Could you check a few things on this drawing? It's one solid part, dimensions in mm from its lowest x, y, z. Give positions to 0.01 mm unless a question says otherwise; leave off trailing zeros. Order: outer loops, then holes, each group sorted by start corner. A loop starts at its lowest first (then second) coordinate and runs counter-clockwise, first axis right, second up. Notation, with made-up numbers: M 59.5,-39 L 110.5,-39 A26 cw 110.5,-7 Z; hole C 17.5,38.5 d2. An arc over 180 degrees is marked long. Use one line per item in the form item = value.
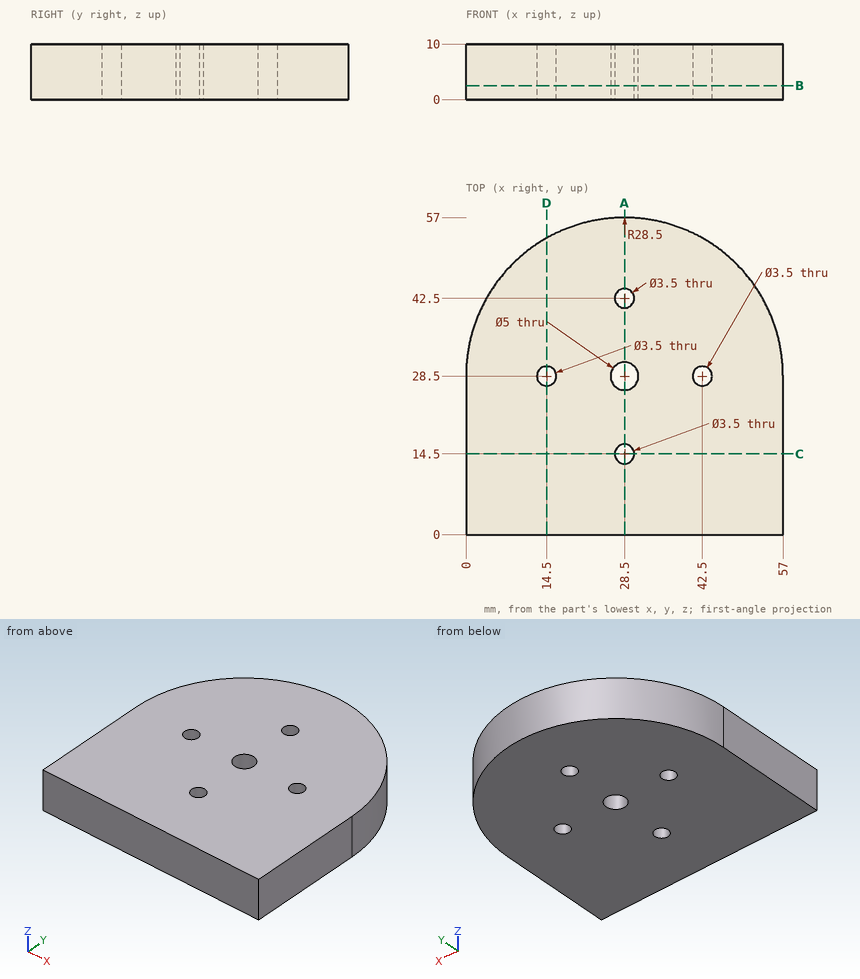
Q1. I want a section at C-C on y = 14.5. Write out the boundary of the cut face in (x, z).
Found:
outline = M 0,0 L 26.75,0 L 26.75,10 L 0,10 Z; M 30.25,0 L 57,0 L 57,10 L 30.25,10 Z
Q2. I need wall thicknesses on L1, parallel to Y at x = 28.5, z = 3.75; L2, parallel to X at y = 30, z = 9; L3, parallel to X at y = 14, z = 4.5. Which ranges of each line are inside material? Lowest first, please.
Found:
L1 = 0 to 12.75, 16.25 to 26, 31 to 40.75, 44.25 to 57
L2 = 0.04 to 13.6, 15.4 to 26.5, 30.5 to 41.6, 43.4 to 56.96
L3 = 0 to 26.82, 30.18 to 57
Q3. I want a section at B-B on z = 2.5. Write out the boundary of the cut face in (x, y), then the cut area to 3 significant figures.
Found:
outline = M 0,0 L 57,0 L 57,28.5 A28.5 ccw 0,28.5 Z; hole C 14.5,28.5 d3.5; hole C 28.5,28.5 d5; hole C 28.5,14.5 d3.5; hole C 28.5,42.5 d3.5; hole C 42.5,28.5 d3.5
area = 2,840 mm²
Q4. I want a section at A-A on x = 28.5. Write out the boundary of the cut face in (y, z).
Found:
outline = M 0,0 L 12.75,0 L 12.75,10 L 0,10 Z; M 16.25,0 L 26,0 L 26,10 L 16.25,10 Z; M 31,0 L 40.75,0 L 40.75,10 L 31,10 Z; M 44.25,0 L 57,0 L 57,10 L 44.25,10 Z
Q5. I want a section at D-D on x = 14.5. Write out the boundary of the cut face in (y, z).
Found:
outline = M 0,0 L 26.75,0 L 26.75,10 L 0,10 Z; M 30.25,0 L 53.32,0 L 53.32,10 L 30.25,10 Z
Q6. I'm going to push flat-ended pins straight in: pin 1 Ø2 at (x, y) = (28.5, 42.5) entering from -Z; pin 2 Ø6 at (x, z) = (12.5, 8) entering from +Y; pin 3 Ø5 at (y, z) = (35, 6.5) entering from -X; pin 4 Ø6 at (x, z) = (45, 9) entering from +Y. Where does each tip first touch, or does it pass through?
Found:
pin_1 = through
pin_2 = 53.86
pin_3 = 0.28
pin_4 = 53.6
